Verification items for the finished model (mm, model axes). Round coordinates to 2 decimals unless told otherwise and drop trailing zeros. Order: outer loops, then holes, each group sorted by start corner. A loop starts at its lowest first (then second) coordinate and runs counter-clockwise, first axis right, second up. Notation, with made-up numbers: M 30,55.25 L 55,55.25 A16 ccw 55,70.25 Z; hole C 49,-3 d9. An arc over 180 degrees is marked long. Use one line per item in the form item = value. Start each with the question number.
Item 1: Go/stop test with a flat-tipped pin: pin 1 Ø1.5 at (y, z) = (-59.5, 2.5) entering from -X. Record where the tip stops, or that it passes through.
Item 2: Thickness scan on probe 1 along Y at (x, z) = (0, 2.35); probe 2 along X at (y, z) = (59, 2.1); probe 3 along Y at (x, z) = (20, 0.8). Record the ranges inside material, lowest first. Write a range as [from, to].
Item 3: Cross-section at C-C on z = 1.05. Count the separate pieces of the cut face and the enclosed holes in it, then the cut area to 3 significant figures.
Item 4: Cross-section at D-D on x = -82.55. Enter the section's corners in (y, z) (3 decimals), then the cut area to 3 significant figures.
Item 5: Cross-section at A-A on x = 0. Enter the section's corners in (y, z) (3 decimals).
Item 6: Cross-section at B-B on y = 6. Enter the section's corners in (x, z) (3 decimals).
from build123d import *

# Parameters (mm, degrees)
SKETCH1_R           = 88.9
SKETCH1_R_2         = 3.96875
SKETCH1_R_3         = 2.38125
SKETCH1_R_4         = 12.7
BOSS_EXTRUDE1_DEPTH = 3.175


with BuildPart() as part:
    # Sketch1 → Boss-Extrude1 (new body)
    with BuildSketch(Plane.XY):
        Circle(SKETCH1_R)
        with Locations((0, 22.225)):
            Circle(SKETCH1_R_2, mode=Mode.SUBTRACT)
        with Locations((19.247414599, -11.1125)):
            Circle(SKETCH1_R_2, mode=Mode.SUBTRACT)
        with Locations((-19.247414599, -11.1125)):
            Circle(SKETCH1_R_2, mode=Mode.SUBTRACT)
        with Locations((0, 82.55)):
            Circle(SKETCH1_R_3, mode=Mode.SUBTRACT)
        with Locations((58.371664787, 58.371664787)):
            Circle(SKETCH1_R_3, mode=Mode.SUBTRACT)
        with Locations((82.55, 0)):
            Circle(SKETCH1_R_3, mode=Mode.SUBTRACT)
        with Locations((58.371664787, -58.371664787)):
            Circle(SKETCH1_R_3, mode=Mode.SUBTRACT)
        with Locations((0, -82.55)):
            Circle(SKETCH1_R_3, mode=Mode.SUBTRACT)
        with Locations((-58.371664787, -58.371664787)):
            Circle(SKETCH1_R_3, mode=Mode.SUBTRACT)
        with Locations((-82.55, 0)):
            Circle(SKETCH1_R_3, mode=Mode.SUBTRACT)
        with Locations((-58.371664787, 58.371664787)):
            Circle(SKETCH1_R_3, mode=Mode.SUBTRACT)
        Circle(SKETCH1_R_4, mode=Mode.SUBTRACT)
    extrude(amount=BOSS_EXTRUDE1_DEPTH)


solid = part.part
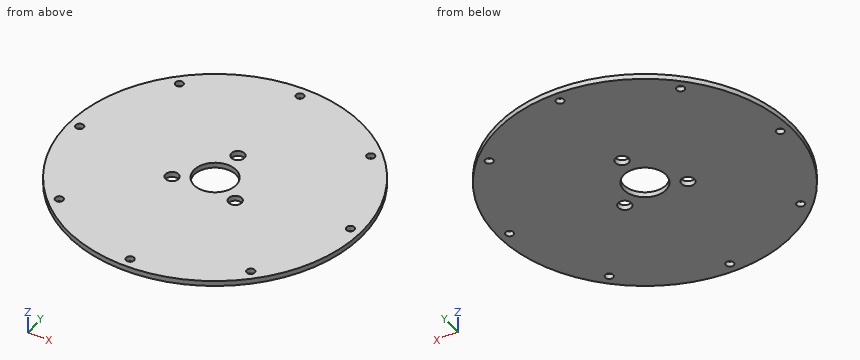
Output values:
q1.pin_1 = -66.72
q2.probe_1 = [-88.9, -84.93], [-80.17, -12.7], [12.7, 18.26], [26.19, 80.17], [84.93, 88.9]
q2.probe_2 = [-66.5, -60.67], [-56.07, 56.07], [60.67, 66.5]
q2.probe_3 = [-86.62, -15.01], [-7.22, 86.62]
q3.separate_pieces = 1
q3.enclosed_holes = 12
q3.area = 24,000 mm2
q4.outline = M -32.996,0 L -2.381,0 L -2.381,3.175 L -32.996,3.175 Z; M 2.381,0 L 32.996,0 L 32.996,3.175 L 2.381,3.175 Z
q4.area = 194 mm2
q5.outline = M -88.9,0 L -84.931,0 L -84.931,3.175 L -88.9,3.175 Z; M -80.169,0 L -12.7,0 L -12.7,3.175 L -80.169,3.175 Z; M 12.7,0 L 18.256,0 L 18.256,3.175 L 12.7,3.175 Z; M 26.194,0 L 80.169,0 L 80.169,3.175 L 26.194,3.175 Z; M 84.931,0 L 88.9,0 L 88.9,3.175 L 84.931,3.175 Z
q6.outline = M -88.697,0 L -11.193,0 L -11.193,3.175 L -88.697,3.175 Z; M 11.193,0 L 88.697,0 L 88.697,3.175 L 11.193,3.175 Z
